```python
from build123d import *

# Parameters (mm, degrees)
SKETCH_1_W          = 71.6
SKETCH_1_H          = 80
SKETCH_1_R          = 2.1
EXTRUDE_1_DEPTH     = 3
SKETCH_2_R          = 1.6
CUT_EXTRUDE_1_DEPTH = 3
SKETCH_3_R          = 15
CUT_EXTRUDE_2_DEPTH = 3
CUT_EXTRUDE_3_DEPTH = 3


with BuildPart() as part:
    # 草图1 → 凸台-拉伸1 (new body)
    with BuildSketch(Plane.XY):
        with Locations((0, -4.2)):
            Rectangle(SKETCH_1_W, SKETCH_1_H)
        with Locations((-29.8, 29.8)):
            Circle(SKETCH_1_R, mode=Mode.SUBTRACT)
        with Locations((29.8, 29.8)):
            Circle(SKETCH_1_R, mode=Mode.SUBTRACT)
        with BuildLine():
            ThreePointArc((8.833273811, -16.153781887), (8.833273811, -18.487234265), (11.166726189, -18.487234265))
            ThreePointArc((11.166726189, -18.487234265), (11.166726189, -16.153781887), (8.833273811, -16.153781887))
        make_face(mode=Mode.SUBTRACT)
        with BuildLine():
            ThreePointArc((-21.166726189, 1.166726189), (-21.166726189, -1.166726189), (-18.833273811, -1.166726189))
            ThreePointArc((-18.833273811, -1.166726189), (-18.833273811, 1.166726189), (-21.166726189, 1.166726189))
        make_face(mode=Mode.SUBTRACT)
        with BuildLine():
            ThreePointArc((8.833273811, 18.487234265), (8.833273811, 16.153781887), (11.166726189, 16.153781887))
            ThreePointArc((11.166726189, 16.153781887), (11.166726189, 18.487234265), (8.833273811, 18.487234265))
        make_face(mode=Mode.SUBTRACT)
    extrude(amount=EXTRUDE_1_DEPTH)

    # 草图2 → 切除-拉伸1 (cut)
    with BuildSketch(Plane.XY.offset(3)):
        with Locations((29.8, -37.2)):
            Circle(SKETCH_2_R)
        with Locations((17.8, -37.2)):
            Circle(SKETCH_2_R)
        with Locations((-17.8, -37.2)):
            Circle(SKETCH_2_R)
        with Locations((-29.8, -37.2)):
            Circle(SKETCH_2_R)
    extrude(amount=-CUT_EXTRUDE_1_DEPTH, mode=Mode.SUBTRACT)

    # 草图3 → 切除-拉伸2 (cut)
    with BuildSketch(Plane.XY.offset(3)):
        Circle(SKETCH_3_R)
    extrude(amount=-CUT_EXTRUDE_2_DEPTH, mode=Mode.SUBTRACT)

    # 草图4 → 切除-拉伸3 (cut)
    with BuildSketch(Plane.XY.offset(3)):
        with BuildLine():
            Line((12, 17.320508076), (12, 16.320508076))
            ThreePointArc((12, 16.320508076), (10, 14.320508076), (8, 16.320508076))
            Line((8, 16.320508076), (8, 17.320508076))
            ThreePointArc((8, 17.320508076), (10, 19.320508076), (12, 17.320508076))
        make_face()
        with BuildLine():
            Line((-18, 0), (-18, -1))
            ThreePointArc((-18, -1), (-20, -3), (-22, -1))
            Line((-22, -1), (-22, 0))
            ThreePointArc((-22, 0), (-20, 2), (-18, 0))
        make_face()
        with BuildLine():
            Line((12, -17.320508076), (12, -18.320508076))
            ThreePointArc((12, -18.320508076), (10, -20.320508076), (8, -18.320508076))
            Line((8, -18.320508076), (8, -17.320508076))
            ThreePointArc((8, -17.320508076), (10, -15.320508076), (12, -17.320508076))
        make_face()
    extrude(amount=-CUT_EXTRUDE_3_DEPTH, mode=Mode.SUBTRACT)


solid = part.part
```
The listing builds one solid part. Answer for the finished solid, in the listing's coordinates (mm). A direction names the side the tool comes from. Give positions to 0.01 mm unless a question says otherwise; leave off trailing zeros. Order: outer loops, then holes, each group sorted by start corner. A loop starts at its lowest first (then second) coordinate and runs counter-clockwise, first axis right, second up. Notation, with made-up numbers: (4.25, 29.25) - (21.25, 29.25) arc R23 cw to (21.25, 63.25) - close; hole circle Ø8 at (48, 13). An arc over 180 degrees is marked (long way). Use one line per item in the form item = value. Start each with the question number.
(1) For faces 5 (the flat face through (-1, 35.8, 1)), 6 (the cylindrical face through (-20, 2, 2)), determine the directions among +Z, -Z, +X, -X, +Y, -Y from which every point of the face is accessible in a straight line to the end or side of a thin tool.
(2) A cutting plane is placed at A-A, the plane x = 29.8. Write down the section's boundary in (y, z), then the cut area to 3 significant figures.
(3) A cutting plane is placed at B-B, the plane y = 9. Write down the section's boundary in (x, z), then the cut area to 3 significant figures.
(4) A cutting plane is placed at C-C, the plane x = 17.8. Write down the section's boundary in (y, z), then the cut area to 3 significant figures.
(5) The mould has two halves that part along X. Classify faces 1 (the cylindrical face through (16.53, -38.17, 1.52)), 2 (the flat face through (35.8, -5, 1)), 3 (the cylindrical face through (-30.073, 31.882, 1.479)), 4 (the flat face through (-1, -44.2, 1)): released by +X, released by -X, zero draft, split by the parting line, or undercut.
(6) Consider line 1 (Y direction, x = 29.8, z = 1); line 2 (Y direction, x = 17.8, z = 1.6); line 3 (Y direction, x = -20, z = 0.8). Determine where each line is inside the solid, lowest interval first. Write a range as from..to.
(7) A cutting plane is placed at D-D, the plane z = 2.05. State how many separate pieces and enclosed holes the cut face has, then the cut area to 3 significant figures.
(8) Flat-ended cylindrical pins translate along their axes: pin 1 Ø3.5 at (x, y) = (17.8, -37.2) entering from -Z; pin 2 Ø3.5 at (x, y) = (-29.8, 29.8) entering from +Z. Find the tip coordinate at first contact, or state that the pin passes through.
Ans:
q1.face_5 = +Z, -Z, +X, -X, +Y
q1.face_6 = +Z, -Z
q2.outline = (-44.2, 0) - (-38.8, 0) - (-38.8, 3) - (-44.2, 3) - close; (-35.6, 0) - (27.7, 0) - (27.7, 3) - (-35.6, 3) - close; (31.9, 0) - (35.8, 0) - (35.8, 3) - (31.9, 3) - close
q2.area = 218 mm^2
q3.outline = (-35.8, 0) - (-12, 0) - (-12, 3) - (-35.8, 3) - close; (12, 0) - (35.8, 0) - (35.8, 3) - (12, 3) - close
q3.area = 143 mm^2
q4.outline = (-44.2, 0) - (-38.8, 0) - (-38.8, 3) - (-44.2, 3) - close; (-35.6, 0) - (35.8, 0) - (35.8, 3) - (-35.6, 3) - close
q4.area = 230 mm^2
q5.face_1 = undercut
q5.face_2 = released by +X
q5.face_3 = undercut
q5.face_4 = zero draft
q6.line_1 = -44.2..-38.8, -35.6..27.7, 31.9..35.8
q6.line_2 = -44.2..-38.8, -35.6..35.8
q6.line_3 = -44.2..-3, 2..35.8
q7.separate_pieces = 1
q7.enclosed_holes = 10
q7.area = 4,910 mm^2
q8.pin_1 = 0
q8.pin_2 = through
